Here's how the part is built. I have some questions about the finished solid (model axes, mm). Face numbers are marked on the shaded views. A direction names the side the tool comes from. Give positions to 0.01 mm unless a question says otherwise; leave off trailing zeros. Write each loop counter-clockwise with the first axis right and the second up, starting at its lowest first coordinate (ties: lowest second). Pieces come first, ordered by that corner, then holes. Notation, with made-up numbers: (2, 14) - (47, 14) arc R31 ccw to (47, 53) - close; hole circle Ø11 at (86.25, 36.25). An arc over 180 degrees is marked (long way). Use a Markdown table: item, result.
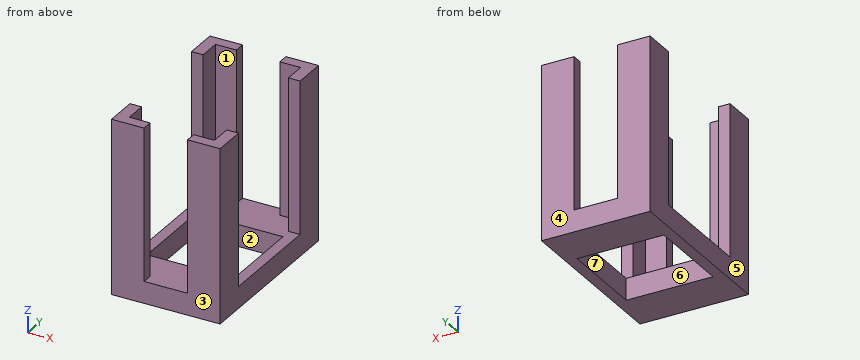
Autodesk Fusion 360 part; units mm, degrees
sketch "スケッチ1" plane through (0, 0, 0) normal (0, 0, 1) x (1, 0, 0)
  line L0 (25, -40) -> (-25, -40)
  line L1 (-25, -40) -> (-25, 40)
  line L2 (-25, 40) -> (25, 40)
  line L3 (25, 40) -> (25, -40)
  line L4 (25, -40) -> (-25, 40) construction
  line L5 (-25, -40) -> (25, 40) construction
  dimension "d1" = 50
  dimension "d2" = 80
extrude "押し出し1" add sketch "スケッチ1" along normal blind 80
sketch "スケッチ2" plane through (0, 0, 80) normal (0, 0, 1) x (-1, 0, 0)
  line L0 (-25, -40) -> (25, -40)
  line L1 (25, -40) -> (25, 40)
  line L2 (25, 40) -> (-25, 40)
  line L3 (-25, 40) -> (-25, -40)
  line L4 (-19.6, 35) -> (19.6, 35)
  line L5 (19.6, 35) -> (19.6, -35)
  line L6 (19.6, -35) -> (-19.6, -35)
  line L7 (-19.6, -35) -> (-19.6, 35)
  line L8 (-19.6, 35) -> (19.6, -35) construction
  line L9 (19.6, 35) -> (-19.6, -35) construction
  dimension "d5" = 39.2
  dimension "d6" = 70
extrude "押し出し2" cut sketch "スケッチ2" against normal blind 70 contours L4 L5 L6 L7
sketch "スケッチ4" plane through (0, 0, 80) normal (0, 0, 1) x (-1, 0, 0)
  line L0 (19.6, 35) -> (19.6, -35)
  line L1 (19.6, -35) -> (-19.6, -35)
  line L2 (-19.6, -35) -> (-19.6, 35)
  line L3 (-19.6, 35) -> (19.6, 35)
  line L4 (-25, -40) -> (25, -40)
  line L5 (25, -40) -> (25, 40)
  line L6 (25, 40) -> (-25, 40)
  line L7 (-25, 40) -> (-25, -40)
  line L8 (-30, 25) -> (30, 25)
  line L9 (30, 25) -> (30, -25)
  line L10 (30, -25) -> (-30, -25)
  line L11 (-30, -25) -> (-30, 25)
  line L12 (-30, 25) -> (30, -25) construction
  line L13 (30, 25) -> (-30, -25) construction
  dimension "d11" = 60
  dimension "d12" = 50
extrude "押し出し4" cut sketch "スケッチ4" against normal blind 70 contours L0 L5 L8 L10 | L2 L7 L8 L10
sketch "スケッチ5" plane through (0, 0, 10) normal (0, 0, 1) x (-1, 0, 0)
  line L0 (-19.6, -35) -> (19.6, -35)
  line L1 (19.6, -35) -> (19.6, -25)
  line L2 (19.6, -25) -> (25, -25)
  line L3 (25, -25) -> (25, 25)
  line L4 (25, 25) -> (19.6, 25)
  line L5 (19.6, 25) -> (19.6, 35)
  line L6 (19.6, 35) -> (-19.6, 35)
  line L7 (-19.6, 35) -> (-19.6, 25)
  line L8 (-19.6, 25) -> (-25, 25)
  line L9 (-25, 25) -> (-25, -25)
  line L10 (-25, -25) -> (-19.6, -25)
  line L11 (-19.6, -25) -> (-19.6, -35)
  line L12 (-20, 20) -> (20, 20)
  line L13 (20, 20) -> (20, -20)
  line L14 (20, -20) -> (-20, -20)
  line L15 (-20, -20) -> (-20, 20)
  line L16 (-20, 20) -> (20, -20) construction
  line L17 (20, 20) -> (-20, -20) construction
extrude "押し出し5" cut sketch "スケッチ5" against normal blind 10 contours L12 L13 L14 L15
sketch "スケッチ6" plane through (0, -40, 0) normal (0, -1, 0) x (1, 0, 0)
  line L0 (-25, 0) -> (25, 0)
  line L1 (25, 0) -> (25, 80)
  line L2 (25, 80) -> (-25, 80)
  line L3 (-25, 80) -> (-25, 0)
  line L4 (-10, 80) -> (10, 80)
  line L5 (10, 80) -> (10, 10)
  line L6 (10, 10) -> (-10, 10)
  line L7 (-10, 10) -> (-10, 80)
extrude "押し出し6" cut sketch "スケッチ6" against normal blind 100 contours L2 L4 L5 L6 L7
Item 1: If we section it at C-C, the plane y = -8.5: Write out the boundary of the cut face in (x, z), plus the area to 3 significant figures.
Values:
| item | result |
|---|---|
| outline | (-25, 0) - (-20, 0) - (-20, 10) - (-25, 10) - close; (20, 0) - (25, 0) - (25, 10) - (20, 10) - close |
| area | 100 mm2 |
Item 2: Thinking about a two-plate mould opening in X: for the marked faces 4, 5, 6 and 7, which applies, +X half, -X half, draft (parallel to the pull), parting line (faces both ways), or undercut?
Values:
| item | result |
|---|---|
| face 4 | draft |
| face 5 | -X half |
| face 6 | undercut |
| face 7 | undercut |
Item 3: I need wall thicknesses on line 1 along Y through (x, z) = (19, 55); line 2 along Y through (x, z) = (-20.5, 23); line 3 along X through (y, z) = (-2.5, 9). Which ranges of each line are inside material? Lowest first, please. Write a range as [from, to].
Values:
| item | result |
|---|---|
| line 1 | y = [-40, -35], [35, 40] |
| line 2 | y = [-40, -25], [25, 40] |
| line 3 | x = [-25, -20], [20, 25] |
Item 4: If we section it at D-D, the plane z = 7: Write out the boundary of the cut face in (x, y).
Values:
| item | result |
|---|---|
| outline | (-25, -40) - (25, -40) - (25, 40) - (-25, 40) - close; hole (-20, -20) - (20, -20) - (20, 20) - (-20, 20) - close |
Item 5: For the marked faces 1, 2 and 3, which set-ups out of +Z, -Z, +X, -X, +Y, -Y let a thin tool reach every point of the face, with its end or its side?
Values:
| item | result |
|---|---|
| face 1 | +Z |
| face 2 | +Z, -Z |
| face 3 | +Z, -Z, +X, -X, -Y |
Item 6: If we section it at A-A, the plane z = 65.5: Write out the boundary of the cut face in (x, y).
Values:
| item | result |
|---|---|
| outline | (-25, -40) - (-10, -40) - (-10, -35) - (-19.6, -35) - (-19.6, -25) - (-25, -25) - close; (-25, 25) - (-19.6, 25) - (-19.6, 35) - (-10, 35) - (-10, 40) - (-25, 40) - close; (10, -40) - (25, -40) - (25, -25) - (19.6, -25) - (19.6, -35) - (10, -35) - close; (10, 35) - (19.6, 35) - (19.6, 25) - (25, 25) - (25, 40) - (10, 40) - close |
Item 7: If we section it at B-B, the plane x = -6: Write out the boundary of the cut face in (y, z).
Values:
| item | result |
|---|---|
| outline | (-40, 0) - (-20, 0) - (-20, 10) - (-40, 10) - close; (20, 0) - (40, 0) - (40, 10) - (20, 10) - close |
